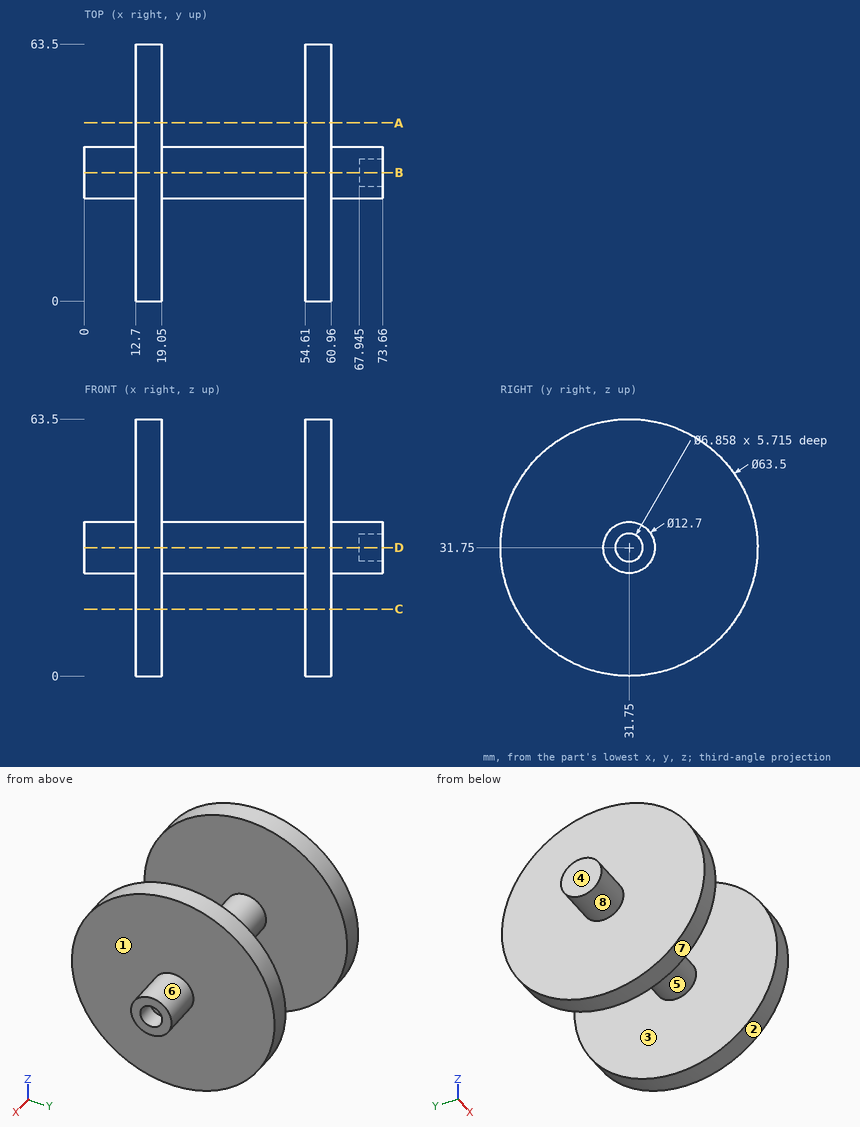
Geometry: see drawing. Coordinates: mm, zero at the bounding-box minimum. A direction names the side the tool comes from. Round coordinates to 2 decimals unless told otherwise and drop trailing zeros. Loops run counter-clockwise (first coordinate to the right, second up) from the corner with the lowest first, then second, coordinate; pieces in that order, holes last. Notation, with made-up numbers: M 72,6.5 L 93,6.5 A16 cw 93,25.5 Z; hole C -27.75,33.5 d5. An arc over 180 degrees is marked long. Use a Markdown table: item, result. Add a question column.
1. Pull-direction query (X, two-part tool) for the marked faces 1, 2 and 3; classes: +X half, -X half, draft (parallel to the pull), parting line (faces both ways), or undercut.
2. Set-up query: the marked faces 4, 5, 6, 7 and 8. Return all of +Z, -Z, +X, -X, +Y, -Y with unobstructed straight access to the full face (end or side cutting, diameter ignored); none if empty.
3. Cut plane A-A, the plane y = 44. Output: boundary loops of the cut face in (x, z).
4. Cut plane C-C, the plane z = 16.5. Output: boundary loops of the cut face in (x, y).
5. Contact query for flat-ended pins moving along their axis: pin 1 (1 mm diameter, centred on x = 15.5, z = 18.5, fed in from +Y); pin 2 (5 mm diameter, centred on y = 56, z = 35, fed in from +X); pin 3 (8 mm diameter, centred on x = 54, y = 52, fed in from +Z). Output: stop coordinate, or through.
6. Cut plane B-B, the plane y = 31.75. Output: boundary loops of the cut face in (x, z) (3 decimals).
7. Ray query, line 1 along X through (y, z) = (29, 10.5); line 2 along Y through (x, z) = (71.2, 31.75); line 3 along Y through (x, z) = (70, 31). Return the intervals inside material, ascending. Write a range as [from, to].
Solution:
| question | item | result |
|---|---|---|
| 1 | face 1 | +X half |
| 1 | face 2 | draft |
| 1 | face 3 | undercut |
| 2 | face 4 | +Z, -Z, -X, +Y, -Y |
| 2 | face 5 | none |
| 2 | face 6 | +X |
| 2 | face 7 | +X, -X |
| 2 | face 8 | -X |
| 3 | outline | M 12.7,2.46 L 19.05,2.46 L 19.05,61.04 L 12.7,61.04 Z; M 54.61,2.46 L 60.96,2.46 L 60.96,61.04 L 54.61,61.04 Z |
| 4 | outline | M 12.7,3.9 L 19.05,3.9 L 19.05,59.6 L 12.7,59.6 Z; M 54.61,3.9 L 60.96,3.9 L 60.96,59.6 L 54.61,59.6 Z |
| 5 | pin 1 | stops at y = 60.83 |
| 5 | pin 2 | stops at x = 60.96 |
| 5 | pin 3 | stops at z = 59 |
| 6 | outline | M 0,25.4 L 12.7,25.4 L 12.7,0 L 19.05,0 L 19.05,25.4 L 54.61,25.4 L 54.61,0 L 60.96,0 L 60.96,25.4 L 73.66,25.4 L 73.66,28.321 L 67.945,28.321 L 67.945,35.179 L 73.66,35.179 L 73.66,38.1 L 60.96,38.1 L 60.96,63.5 L 54.61,63.5 L 54.61,38.1 L 19.05,38.1 L 19.05,63.5 L 12.7,63.5 L 12.7,38.1 L 0,38.1 Z |
| 7 | line 1 | x = [12.7, 19.05], [54.61, 60.96] |
| 7 | line 2 | y = [25.4, 28.32], [35.18, 38.1] |
| 7 | line 3 | y = [25.44, 28.4], [35.1, 38.06] |
